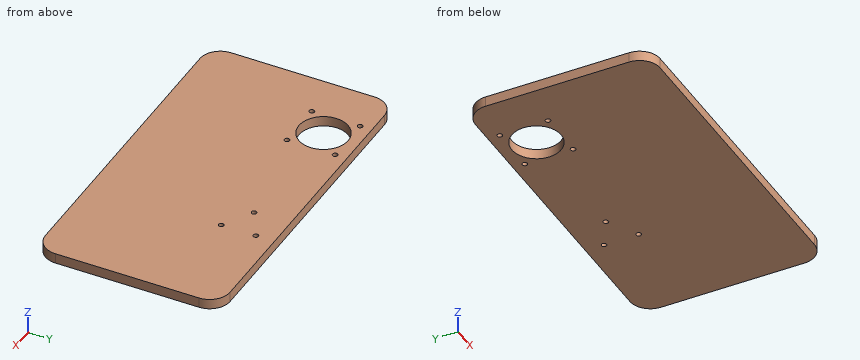
```python
from build123d import *

# Parameters (mm, degrees)
SKETCH_W   = 330
SKETCH_H   = 180
SKETCH_R   = 2.5
SKETCH_R_2 = 24
PAD_DEPTH  = 10
FILLET_R   = 20


with BuildPart() as part:
    # Sketch → Pad (new body)
    with BuildSketch(Plane.XY):
        with Locations((98, -55)):
            Rectangle(SKETCH_W, SKETCH_H)
        with Locations((23.5, 23.5)):
            Circle(SKETCH_R, mode=Mode.SUBTRACT)
        with Locations((-23.5, 23.5)):
            Circle(SKETCH_R, mode=Mode.SUBTRACT)
        with Locations((-23.5, -23.5)):
            Circle(SKETCH_R, mode=Mode.SUBTRACT)
        with Locations((23.5, -23.5)):
            Circle(SKETCH_R, mode=Mode.SUBTRACT)
        Circle(SKETCH_R_2, mode=Mode.SUBTRACT)
        with Locations((159.75, 16.887495)):
            Circle(SKETCH_R, mode=Mode.SUBTRACT)
        with Locations((130.5, 0)):
            Circle(SKETCH_R, mode=Mode.SUBTRACT)
        with Locations((159.75, -16.887495)):
            Circle(SKETCH_R, mode=Mode.SUBTRACT)
    extrude(amount=PAD_DEPTH)

    # Fillet
    fillet_edges = [part.edges().sort_by_distance(p)[0] for p in [
        (-67, -145, 5),
        (263, -145, 5),
        (263, 35, 5),
        (-67, 35, 5),
    ]]
    fillet(fillet_edges, radius=FILLET_R)


solid = part.part
```
Geometry: final body of the model. Coordinates: model frame, mm. Round coordinates to 2 decimals unless told otherwise and drop trailing zeros. Order: outer loops, then holes, each group sorted by start corner. A loop starts at its lowest first (then second) coordinate and runs counter-clockwise, first axis right, second up. Notation, with made-up numbers: (2.25, 64.25) - (20.25, 64.25) arc R19 cw to (20.25, 68.25) - close; hole circle Ø3 at (-12, -12). An arc over 180 degrees is marked (long way). Write item = value, one per line. Start each with the question number.
Q1. Pin query (flat end, axial travel): pin 1 (1.5 mm diameter, centred on y = -126.5, z = 2, fed in from +X); pin 2 (1.5 mm diameter, centred on x = -24, y = -117, fed in from -Z). Return the tip coordinate at first contact, or that it passes through.
Q2. Ray query, line 1 (Y direction, x = 159.75, z = 4.25); line 2 (Y direction, x = 130, z = 2.25); line 3 (X direction, y = -18, z = 3.75). Return the intervals inside material, ascending. Write a range as from..to.
Q3. Cut plane B-B on z = 6.5. Give the number of separate pieces and of enclosed holes in the cut face, and give its area (3 significant figures).
Q4. Cut plane A-A on x = 0. Return the cut outline in (y, z), and give its area (3 significant figures).
Outcome:
q1.pin_1 = 262.99
q1.pin_2 = 0
q2.line_1 = -145..-19.39, -14.39..14.39, 19.39..35
q2.line_2 = -145..-2.45, 2.45..35
q2.line_3 = -67..-15.87, 15.87..157.51, 161.99..263
q3.separate_pieces = 1
q3.enclosed_holes = 8
q3.area = 57,100 mm^2
q4.outline = (-145, 0) - (-24, 0) - (-24, 10) - (-145, 10) - close; (24, 0) - (35, 0) - (35, 10) - (24, 10) - close
q4.area = 1,320 mm^2
